```python
from build123d import *

# Parameters (mm, degrees)
ESQUISSE2_R             = 16
BOSS_EXTRU_1_DEPTH      = 8
ENL_V_MAT_EXTRU_1_DEPTH = 5
ESQUISSE3_R             = 6
ENL_V_MAT_EXTRU_2_DEPTH = 25


with BuildPart() as part:
    # Esquisse2 → Boss.-Extru.1 (new body)
    with BuildSketch(Plane(origin=(0, 0, 0), x_dir=(1, 0, 0), z_dir=(0, 1, 0))):
        with Locations(Location((0, 0, 0), (0, 0, 270))):
            Circle(ESQUISSE2_R)
    extrude(amount=BOSS_EXTRU_1_DEPTH)

    # Esquisse1 → Enlèv. mat.-Extru.1 (cut)
    with BuildSketch(Plane(origin=(0, 0, 0), x_dir=(1, 0, 0), z_dir=(0, 1, 0))):
        with BuildLine():
            Line((-5, 9), (5, 9))
            ThreePointArc((5, 9), (14, 0), (5, -9))
            Line((5, -9), (-5, -9))
            ThreePointArc((-5, -9), (-14, 0), (-5, 9))
        make_face()
    extrude(amount=ENL_V_MAT_EXTRU_1_DEPTH, mode=Mode.SUBTRACT)

    # Esquisse3 → Enlèv. mat.-Extru.2 (cut, through all)
    with BuildSketch(Plane(origin=(0, 8, 0), x_dir=(1, 0, 0), z_dir=(0, 1, 0))):
        with Locations(Location((0, 0, 0), (0, 0, 270))):
            Circle(ESQUISSE3_R)
    extrude(amount=-ENL_V_MAT_EXTRU_2_DEPTH, mode=Mode.SUBTRACT)


solid = part.part
```
The model under review builds one solid part; all positions refer to its coordinate system, in mm. A direction names the side the tool comes from. Round coordinates to 2 decimals unless told otherwise and drop trailing zeros. Write each loop counter-clockwise with the first axis right and the second up, starting at its lowest first coordinate (ties: lowest second). Pieces come first, ordered by that corner, then holes. Notation, with made-up numbers: (14, 51) - (70, 51) arc R31 cw to (70, 77) - close; hole circle Ø4 at (-7, -10). An arc over 180 degrees is marked (long way). One line per question, with ' | ' between items.
Item 1: Add section D-D, the plane x = 11. Give the boundary of the cut face in (y, z).
Resolved:
outline: (0, -11.62) - (8, -11.62) - (8, 11.62) - (0, 11.62) - (0, 6.71) - (5, 6.71) - (5, -6.71) - (0, -6.71) - close
Item 2: For P1, Ø2, axis at y = 3.5, z = -1.5, coming from the +X side; P2, Ø2.5, axis at x = 2, y = 3.5, coming from the +Z side; P3, Ø10, axis at x = -10, z = -7.5, coming from the -Y side, all flat-tipped, find the tip position at first contact; note any pin that passes through.
Resolved:
P1: stops at x = 15.99 | P2: stops at z = 15.98 | P3: stops at y = 0
Item 3: For faces 1 (the face through (-6, 5, 2)), 2 (the face through (0, 0, 10)), list the 3-axis set-ups (+Z, -Z, +X, -X, +Y, -Y) from which the entire face can be reached by the end or side of a thin tool; tool diameter is ignored.
Resolved:
face 1: -Y | face 2: +Z, -Z, +X, -X, -Y
Item 4: Add section B-B, the plane z = 2.5. Give the boundary of the cut face in (x, y).
Resolved:
outline: (-15.8, 0) - (-13.65, 0) - (-13.65, 5) - (-5.45, 5) - (-5.45, 8) - (-15.8, 8) - close; (5.45, 5) - (13.65, 5) - (13.65, 0) - (15.8, 0) - (15.8, 8) - (5.45, 8) - close
Item 5: Add section A-A, the plane x = 0. Give the boundary of the cut face in (y, z), then the cut area to 3 significant figures.
Resolved:
outline: (0, -16) - (8, -16) - (8, -6) - (5, -6) - (5, -9) - (0, -9) - close; (0, 9) - (5, 9) - (5, 6) - (8, 6) - (8, 16) - (0, 16) - close | area: 130 mm2
Item 6: Add section C-C, the plane y = 1. Give the boundary of the cut face in (x, z).
Resolved:
outline: circle Ø32 at (0, 0); hole (-5, -9) - (5, -9) arc R9 ccw to (5, 9) - (-5, 9) arc R9 ccw to start
Item 7: The part is to be moulded in two halves that separate along X. For faces 3 (the face through (0, 8, 7)), 4 (the face through (0, 2, 9)), 5 (the face through (-15.62, 3.94, -3.47)), say which applies: pulls with the +X half, pulls with the -X half, needs draft (parallel to the pull), parting line crosses it, or undercut.
Resolved:
face 3: needs draft | face 4: undercut | face 5: parting line crosses it
Item 8: To check wall thickness, follow probe 1 along X at (y, z) = (6.7, 0); probe 2 along Y at (x, z) = (7.5, 0); probe 3 along X at (y, z) = (5.75, -3). State the ranges of each line that lie inside material, in increasing order.
Resolved:
probe 1: x = -16 to -6, 6 to 16 | probe 2: y = 5 to 8 | probe 3: x = -15.72 to -5.2, 5.2 to 15.72
